```python
from build123d import *

# Parameters (mm, degrees)
SKETCH1_W           = 40
SKETCH1_H           = 55
SKETCH1_R           = 5.207
SKETCH1_R_2         = 7.6
BOSS_EXTRUDE1_DEPTH = 40
SKETCH1_3_R         = 11.1125
SKETCH1_3_R_2       = 5.207
CUT_EXTRUDE1_DEPTH  = 6
BOSS_EXTRUDE3_DEPTH = 16
CHAMFER1_SIZE       = 1
CUT_EXTRUDE2_START  = 6
SKETCH2_R           = 2.05
CUT_EXTRUDE2_DEPTH  = 6
SKETCH3_R           = 2.05
CUT_EXTRUDE3_DEPTH  = 6
SKETCH6_R           = 2.05
CUT_EXTRUDE5_DEPTH  = 7
FILLET2_R           = 3.5
BOSS_EXTRUDE2_DEPTH = 10
CHAMFER4_SIZE       = 1
FILLET3_R           = 3


with BuildPart() as part:
    # Sketch1 → Boss-Extrude1 (new body)
    with BuildSketch(Plane(origin=(0, 0, 0), x_dir=(0, 0, -1), z_dir=(1, 0, 0))):
        Rectangle(SKETCH1_W, SKETCH1_H)
        with Locations((0, 12.5)):
            Circle(SKETCH1_R, mode=Mode.SUBTRACT)
        with Locations((0, -12.5)):
            Circle(SKETCH1_R_2, mode=Mode.SUBTRACT)
    extrude(amount=BOSS_EXTRUDE1_DEPTH)

    # Sketch1<3> → Cut-Extrude1 (cut)
    with BuildSketch(Plane(origin=(0, 0, 0), x_dir=(0, 0, -1), z_dir=(1, 0, 0))):
        with Locations((0, 12.5)):
            Circle(SKETCH1_3_R)
        with Locations((0, 12.5)):
            Circle(SKETCH1_3_R_2, mode=Mode.SUBTRACT)
    extrude(amount=CUT_EXTRUDE1_DEPTH, mode=Mode.SUBTRACT)

    # Sketch1<4> → Boss-Extrude3 (add)
    with BuildSketch(Plane(origin=(0, 0, 0), x_dir=(0, 0, -1), z_dir=(1, 0, 0))):
        with BuildLine():
            ThreePointArc((7.6, -12.5), (5.374011537, -7.125988463), (0, -4.9))
            ThreePointArc((0, -4.9), (-5.374011537, -17.874011537), (7.6, -12.5))
        make_face()
        with BuildLine():
            ThreePointArc((4.5, -12.5), (-3.181980515, -15.681980515), (0, -8))
            ThreePointArc((0, -8), (3.181980515, -9.318019485), (4.5, -12.5))
        make_face(mode=Mode.SUBTRACT)
    extrude(amount=BOSS_EXTRUDE3_DEPTH)

    # Chamfer1
    chamfer1_edges = [part.edges().sort_by_distance(p)[0] for p in [
        (6, 12.5, 5.207),
        (0, 12.5, 11.1125),
        (40, 12.5, 5.207),
        (40, -12.5, 7.6),
    ]]
    chamfer(chamfer1_edges, length=CHAMFER1_SIZE)

    # Sketch2 → Cut-Extrude2 (cut)
    with BuildSketch(Plane(origin=(0, 0, 0), x_dir=(0, 0, -1), z_dir=(1, 0, 0)).offset(CUT_EXTRUDE2_START)):
        with Locations(Location((0, 4.65475, 0), (0, 0, 122.182106199))):
            Circle(SKETCH2_R)
        with Locations(Location((-7.84525, 12.5, 0), (0, 0, 327.817891972))):
            Circle(SKETCH2_R)
        with Locations(Location((0, 20.34525, 0), (0, 0, 237.817891972))):
            Circle(SKETCH2_R)
        with Locations(Location((7.84525, 12.5, 0), (0, 0, 212.182106199))):
            Circle(SKETCH2_R)
    extrude(amount=CUT_EXTRUDE2_DEPTH, mode=Mode.SUBTRACT)

    # Sketch3 → Cut-Extrude3 (cut)
    with BuildSketch(Plane(origin=(0, 27.5, 0), x_dir=(1, 0, 0), z_dir=(0, 1, 0))):
        with Locations(Location((12.5, 10, 0), (0, 0, 270))):
            Circle(SKETCH3_R)
        with Locations(Location((27.5, 10, 0), (0, 0, 270))):
            Circle(SKETCH3_R)
        with Locations(Location((12.5, -10, 0), (0, 0, 270))):
            Circle(SKETCH3_R)
        with Locations(Location((27.5, -10, 0), (0, 0, 270))):
            Circle(SKETCH3_R)
    extrude(amount=-CUT_EXTRUDE3_DEPTH, mode=Mode.SUBTRACT)

    # Sketch6 → Cut-Extrude5 (cut)
    with BuildSketch(Plane(origin=(0, 0, -20), x_dir=(-1, 0, 0), z_dir=(0, 0, -1))):
        with Locations((-27.5, 17.5)):
            Circle(SKETCH6_R)
        with Locations((-12.5, 17.5)):
            Circle(SKETCH6_R)
        with Locations((-27.5, -2.5)):
            Circle(SKETCH6_R)
        with Locations((-12.5, -2.5)):
            Circle(SKETCH6_R)
    cut_extrude5 = extrude(amount=-CUT_EXTRUDE5_DEPTH, mode=Mode.SUBTRACT)

    # Mirror1: Cut-Extrude5 across plane
    add(cut_extrude5.mirror(Plane.XY), mode=Mode.SUBTRACT)

    # Chamfer3: read off the stored shape, not the designer's step
    # Chamfer3: loft between two sections, ruled curve by curve
    chamfer3_from = [
        Edge.make_three_point_arc((15, -12.5, -4.5), (15, -8, 0), (15, -12.5, 4.5)),
        Edge.make_three_point_arc((15, -12.5, 4.5), (15, -17, 0), (15, -12.5, -4.5)),
    ]
    chamfer3_to = [
        Edge.make_three_point_arc((16, -12.5, -5.5), (16, -7, 0), (16, -12.5, 5.5)),
        Edge.make_three_point_arc((16, -12.5, 5.5), (16, -18, 0), (16, -12.5, -5.5)),
    ]
    chamfer3 = Solid(Shell([*[Face.make_surface_from_curves(chamfer3_from[k], chamfer3_to[k]) for k in range(2)], Face(Wire(chamfer3_from)), Face(Wire(chamfer3_to))]))
    add(chamfer3, mode=Mode.SUBTRACT)

    # Chamfer3 2: loft between two sections, ruled curve by curve
    chamfer3_2_from = [
        Edge.make_three_point_arc((1, -12.5, -4.5), (1, -17, 0), (1, -12.5, 4.5)),
        Edge.make_three_point_arc((1, -12.5, 4.5), (1, -8, 0), (1, -12.5, -4.5)),
    ]
    chamfer3_2_to = [
        Edge.make_three_point_arc((0, -12.5, -5.5), (0, -18, 0), (0, -12.5, 5.5)),
        Edge.make_three_point_arc((0, -12.5, 5.5), (0, -7, 0), (0, -12.5, -5.5)),
    ]
    chamfer3_2 = Solid(Shell([*[Face.make_surface_from_curves(chamfer3_2_from[k], chamfer3_2_to[k]) for k in range(2)], Face(Wire(chamfer3_2_from)), Face(Wire(chamfer3_2_to))]))
    add(chamfer3_2, mode=Mode.SUBTRACT)

    # Chamfer3 3: loft between two sections, ruled curve by curve
    chamfer3_3_from = [
        Edge.make_three_point_arc((7, 14.011711483, 6.460609833), (7, 11.115359819, 6.33353853), (7, 10.988288542, 9.229890194)),
        Edge.make_three_point_arc((7, 10.988288542, 9.229890194), (7, 13.884640208, 9.356961446), (7, 14.011711483, 6.460609833)),
    ]
    chamfer3_3_to = [
        Edge.make_three_point_arc((6, 14.749131718, 5.785175605), (6, 10.439925585, 5.5961183), (6, 10.250868319, 9.905324435)),
        Edge.make_three_point_arc((6, 10.250868319, 9.905324435), (6, 14.560074456, 10.094381663), (6, 14.749131718, 5.785175605)),
    ]
    chamfer3_3 = Solid(Shell([*[Face.make_surface_from_curves(chamfer3_3_from[k], chamfer3_3_to[k]) for k in range(2)], Face(Wire(chamfer3_3_from)), Face(Wire(chamfer3_3_to))]))
    add(chamfer3_3, mode=Mode.SUBTRACT)

    # Chamfer3 4: loft between two sections, ruled curve by curve
    chamfer3_4_from = [
        Edge.make_three_point_arc((7, 18.960609833, -1.511711483), (7, 18.83353853, 1.384640181), (7, 21.729890194, 1.511711458)),
        Edge.make_three_point_arc((7, 21.729890194, 1.511711458), (7, 21.856961446, -1.384640208), (7, 18.960609833, -1.511711483)),
    ]
    chamfer3_4_to = [
        Edge.make_three_point_arc((6, 18.285175605, -2.249131718), (6, 18.0961183, 2.060074415), (6, 22.405324435, 2.249131681)),
        Edge.make_three_point_arc((6, 22.405324435, 2.249131681), (6, 22.594381663, -2.060074456), (6, 18.285175605, -2.249131718)),
    ]
    chamfer3_4 = Solid(Shell([*[Face.make_surface_from_curves(chamfer3_4_from[k], chamfer3_4_to[k]) for k in range(2)], Face(Wire(chamfer3_4_from)), Face(Wire(chamfer3_4_to))]))
    add(chamfer3_4, mode=Mode.SUBTRACT)

    # Chamfer3 5: loft between two sections, ruled curve by curve
    chamfer3_5_from = [
        Edge.make_three_point_arc((7, 10.988288517, -6.460609833), (7, 13.884640181, -6.33353853), (7, 14.011711458, -9.229890194)),
        Edge.make_three_point_arc((7, 14.011711458, -9.229890194), (7, 11.115359792, -9.356961446), (7, 10.988288517, -6.460609833)),
    ]
    chamfer3_5_to = [
        Edge.make_three_point_arc((6, 10.250868282, -5.785175605), (6, 14.560074415, -5.5961183), (6, 14.749131681, -9.905324435)),
        Edge.make_three_point_arc((6, 14.749131681, -9.905324435), (6, 10.439925544, -10.094381663), (6, 10.250868282, -5.785175605)),
    ]
    chamfer3_5 = Solid(Shell([*[Face.make_surface_from_curves(chamfer3_5_from[k], chamfer3_5_to[k]) for k in range(2)], Face(Wire(chamfer3_5_from)), Face(Wire(chamfer3_5_to))]))
    add(chamfer3_5, mode=Mode.SUBTRACT)

    # Chamfer3 6: loft between two sections, ruled curve by curve
    chamfer3_6_from = [
        Edge.make_three_point_arc((7, 6.039390167, 1.511711483), (7, 6.16646147, -1.384640181), (7, 3.270109806, -1.511711458)),
        Edge.make_three_point_arc((7, 3.270109806, -1.511711458), (7, 3.143038554, 1.384640208), (7, 6.039390167, 1.511711483)),
    ]
    chamfer3_6_to = [
        Edge.make_three_point_arc((6, 6.714824395, 2.249131718), (6, 6.9038817, -2.060074415), (6, 2.594675565, -2.249131681)),
        Edge.make_three_point_arc((6, 2.594675565, -2.249131681), (6, 2.405618337, 2.060074456), (6, 6.714824395, 2.249131718)),
    ]
    chamfer3_6 = Solid(Shell([*[Face.make_surface_from_curves(chamfer3_6_from[k], chamfer3_6_to[k]) for k in range(2)], Face(Wire(chamfer3_6_from)), Face(Wire(chamfer3_6_to))]))
    add(chamfer3_6, mode=Mode.SUBTRACT)

    # Fillet2
    fillet2_edges = [part.edges().sort_by_distance(p)[0] for p in [
        (40, 0, -20),
        (40, 0, 20),
        (0, 0, 20),
        (0, 0, -20),
    ]]
    fillet(fillet2_edges, radius=FILLET2_R)

    # Sketch5 → Boss-Extrude2 (add)
    with BuildSketch(Plane.XZ.offset(27.5)):
        with BuildLine():
            Line((16.4, 18.68), (16.4, 8.4))
            Line((16.4, 8.4), (23.6, 8.4))
            Line((23.6, 8.4), (23.6, 18.68))
            ThreePointArc((23.6, 18.68), (23.761942699, 19.408599647), (24.2172761, 20))
            Line((24.2172761, 20), (15.7827239, 20))
            ThreePointArc((15.7827239, 20), (16.238057301, 19.408599647), (16.4, 18.68))
        make_face()
        with BuildLine():
            ThreePointArc((1.32, 3.6), (0.591400353, 3.761942699), (0, 4.2172761))
            Line((0, 4.2172761), (0, -4.2172761))
            ThreePointArc((0, -4.2172761), (0.591400353, -3.761942699), (1.32, -3.6))
            Line((1.32, -3.6), (11.6, -3.6))
            Line((11.6, -3.6), (11.6, 3.6))
            Line((11.6, 3.6), (1.32, 3.6))
        make_face()
        with BuildLine():
            Line((40, -4.2172761), (40, 4.2172761))
            ThreePointArc((40, 4.2172761), (39.408599647, 3.761942699), (38.68, 3.6))
            Line((38.68, 3.6), (28.4, 3.6))
            Line((28.4, 3.6), (28.4, -3.6))
            Line((28.4, -3.6), (38.68, -3.6))
            ThreePointArc((38.68, -3.6), (39.408599647, -3.761942699), (40, -4.2172761))
        make_face()
        with BuildLine():
            ThreePointArc((16.4, -18.68), (16.238057301, -19.408599647), (15.7827239, -20))
            Line((15.7827239, -20), (24.2172761, -20))
            ThreePointArc((24.2172761, -20), (23.761942699, -19.408599647), (23.6, -18.68))
            Line((23.6, -18.68), (23.6, -8.4))
            Line((23.6, -8.4), (16.4, -8.4))
            Line((16.4, -8.4), (16.4, -18.68))
        make_face()
    extrude(amount=BOSS_EXTRUDE2_DEPTH)

    # Chamfer4
    chamfer4_edges = [part.edges().sort_by_distance(p)[0] for p in [
        (29.55, -2.5, -20),
        (14.55, -2.5, -20),
        (29.55, 17.5, -20),
        (14.55, 17.5, 20),
        (29.55, -2.5, 20),
        (14.55, -2.5, 20),
        (29.55, 17.5, 20),
        (27.5, 27.5, -12.05),
        (12.5, 27.5, 7.95),
        (27.5, 27.5, 7.95),
        (12.5, 27.5, -12.05),
        (14.55, 17.5, -20),
    ]]
    chamfer(chamfer4_edges, length=CHAMFER4_SIZE)

    # Fillet3
    fillet3_edges = [part.edges().sort_by_distance(p)[0] for p in [
        (16.4, -32.5, 8.4),
        (23.6, -32.5, 8.4),
        (11.6, -32.5, -3.6),
        (11.6, -32.5, 3.6),
        (28.4, -32.5, 3.6),
        (28.4, -32.5, -3.6),
        (23.6, -32.5, -8.4),
        (16.4, -32.5, -8.4),
    ]]
    fillet(fillet3_edges, radius=FILLET3_R)


solid = part.part
```
Build history of the part. All positions in model axes, mm. A direction names the side the tool comes from. Give positions to 0.01 mm unless a question says otherwise; leave off trailing zeros. Loops run counter-clockwise (first coordinate to the right, second up) from the corner with the lowest first, then second, coordinate; pieces in that order, holes last. Notation, with made-up numbers: (2, 57) -> (47, 57) arc R12 cw to (47, 64) -> close; hole circle Ø6 at (-22, 43). An arc over 180 degrees is marked (long way). One line per question, with ' | ' between items. Start each with the question number.
1) Two-plate mould, pull along X, no slides. Class faces 1 (the cylindrical face through (14.55, -2.41, 16.04)), 2 (the flat face through (16.4, -32, 15)), 3 (the cylindrical face through (38.95, 0.39, 19)), 4 (the cylindrical face through (28.9, 24, 8.5)): released by +X, released by -X, zero draft, split by the parting line, or undercut.
2) Cut at A-A (x = 34.5). Give the cut face in (y, z).
3) 3-axis set-ups, long thin cutter, end or side, ignore diameter. For faces 5 (the cylindrical face through (29.26, -32.57, 2.7)), 6 (the flat face through (16.4, -32, -15)), 7 (the cylindrical face through (29.55, -2.41, 16.04)), 8 (the flat face through (12, 5, 0)), 9 (the cylindrical face through (14.55, 17.59, -16.04)): which of +Z, -Z, +X, -X, +Y, -Y reach the whole face in a straight line?
4) Cut at C-C (x = 27.5). Count the separate pieces of the cut face and the enclosed holes in it, plus the area to 3 significant figures.
5) Pin check, flat tips, straight feed: pin 1 (3.5 mm diameter, centred on x = 27.5, y = -2.5, fed in from -Z); pin 2 (3.5 mm diameter, centred on x = 27.5, z = -10, fed in from -Y); pin 3 (20 mm diameter, centred on y = 12.5, z = 0, fed in from -X). Stop position of each tip, or through.
6) Probe L1, parallel to Y at x = 27.5, z = -17.65; L2, parallel to Y at x = 22.5, z = 4; L3, parallel to X at y = 17, z = 15. List the from-to ranges inside material, lowest first.
Return value:
1) face 1: undercut | face 2: released by -X | face 3: released by +X | face 4: undercut
2) outline: (-37.5, -3.6) -> (-27.5, -3.6) -> (-27.5, -20) -> (27.5, -20) -> (27.5, 20) -> (-27.5, 20) -> (-27.5, 3.6) -> (-37.5, 3.6) -> close; hole circle Ø15.2 at (-12.5, 0); hole circle Ø10.41 at (12.5, 0)
3) face 5: +Z, -Y | face 6: -X, -Y | face 7: +Z | face 8: -X | face 9: -Z
4) separate pieces: 1 | enclosed holes: 2 | area: 1,760 mm^2
5) pin 1: z = -13 | pin 2: y = -27.5 | pin 3: x = 6
6) L1: -27.5 to -4.55, -0.45 to 15.45, 19.55 to 27.5 | L2: -27.5 to -18.96, -6.04 to 9.17, 15.83 to 27.5 | L3: 0 to 10.51, 14.49 to 25.51, 29.49 to 40
